Can you work these out from the model? Positions are in its coordinate system, mm. Coordinates: 2 decimals unless noted, no trailing zeros. Write each loop counter-clockwise with the first axis right and the second up, starting at its lowest first coordinate (ties: lowest second). Pieces come first, ordered by that corner, then holes. Notation, with made-up numbers: (62, 55) -> (76, 55) arc R33 ccw to (76, 83) -> close; hole circle Ø11 at (-20, 66.25). An arc over 180 degrees is marked (long way). Use one line per item in the form item = value.
```python
from build123d import *

# Parameters (mm, degrees)
SKETCH_1_R          = 2
EXTRUDE_1_DEPTH     = 18
CUT_EXTRUDE_START   = -7
SKETCH_2_R          = 2
SKETCH_2_R_2        = 1.9
CUT_EXTRUDE_1_DEPTH = 0.5
FILLET_1_R          = 0.1


with BuildPart() as part:
    # 草图1 → 凸台-拉伸1 (new body)
    with BuildSketch(Plane(origin=(0, 0, 0), x_dir=(0, 0, -1), z_dir=(1, 0, 0))):
        Circle(SKETCH_1_R)
    extrude(amount=EXTRUDE_1_DEPTH)

    # 草图2 → 切除-拉伸1 (cut)
    with BuildSketch(Plane(origin=(18, 0, 0), x_dir=(0, 0, -1), z_dir=(1, 0, 0)).offset(CUT_EXTRUDE_START)):
        Circle(SKETCH_2_R)
        Circle(SKETCH_2_R_2, mode=Mode.SUBTRACT)
    cut_extrude_1 = extrude(amount=CUT_EXTRUDE_1_DEPTH, mode=Mode.SUBTRACT)

    # 镜向1: 切除-拉伸1 across plane
    add(cut_extrude_1.mirror(Plane(origin=(9, 0, 0), x_dir=(0, 0, 1), z_dir=(1, 0, 0))), mode=Mode.SUBTRACT)

    # 圆角1
    fillet_1_edges = [part.edges().sort_by_distance(p)[0] for p in [
        (6.5, 0, 1.9),
        (7, 0, 1.9),
        (11, 0, 1.9),
        (11.5, 0, 1.9),
    ]]
    fillet(fillet_1_edges, radius=FILLET_1_R - 0.0001)  # a hair under: the kernel refuses the full size


solid = part.part
```
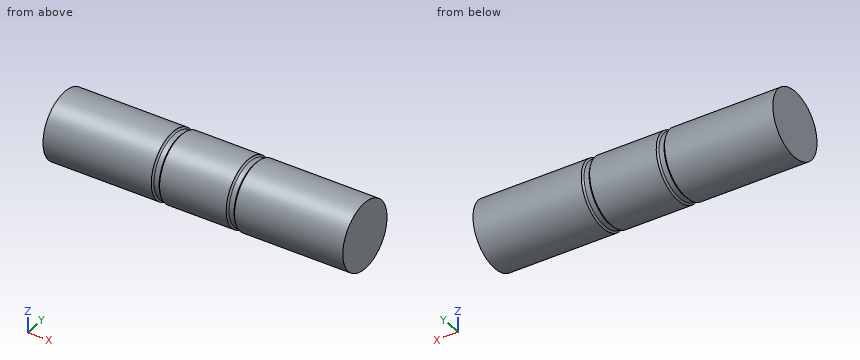
Q1. Suppose I cut it at A-A (x = 15.75). Write out the boundary of the cut face in (y, z), then the cut area to 3 significant figures.
Return value:
outline = circle Ø4 at (0, 0)
area = 12.6 mm2
Q2. Will this pin go through, and if not, where does the flat tip stop? pin 1 (1 mm diameter, centred on x = 15.5, z = -1.5, fed in from -Y).
Return value:
pin_1 = -1.73
Q3. If I drill on line 1 (X direction, y = -1.8, z = -0.8); line 2 (Z direction, x = 6.25, y = 0.1); line 3 (Y direction, x = 12.5, z = 1.2), over which ranges is the centre line in solid material (lowest first)? Write a range as from..to.
Return value:
line_1 = 0..6.5, 7..11, 11.5..18
line_2 = -2..2
line_3 = -1.6..1.6
